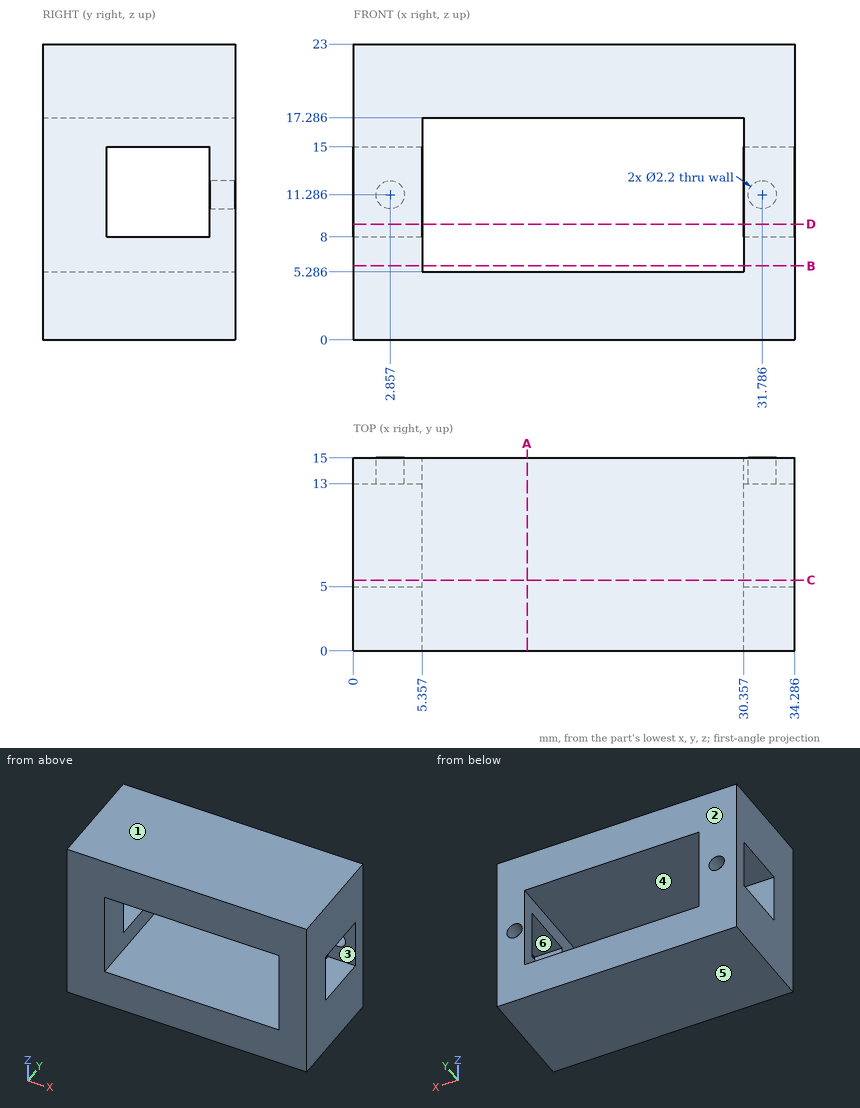
Design review of the part shown in the three views and the two pictorial views. Dimensions are in mm from the part's minimum x, y and z. A direction names the side the tool comes from. Round coordinates to 2 decimals unless told otherwise and drop trailing zeros. Loops run counter-clockwise (first coordinate to the right, second up) from the corner with the lowest first, then second, coordinate; pieces in that order, holes last. Notation, with made-up numbers: (-0.75, -38) -> (10.25, -38) arc R22 ccw to (10.25, -30) -> close; hole circle Ø2 at (14, -29). An arc over 180 degrees is marked (long way). Use one line per item in the form item = value. Start each with the question number.
Q1. For pin 1 Ø1.8 at (x, z) = (31.79, 11.29) entering from +Y, flat-tipped, find the tip position at first contact; note if it passes through.
Q2. Wall thickness on line 1 along Z through (x, y) = (14, 7.75); line 2 along Z through (x, y) = (33.5, 12.25); line 3 along X through (y, z) = (10, 15.75): over which ranges is each line inside the solid? List them lowest first. Write a range as [from, to].
Q3. We need section D-D on z = 9. Give the boundary of the cut face in (x, y), then the cut area to 3 significant figures.
Q4. Draft analysis for pull direction Y (two halves, no side actions). For the marked faces 1, 2 and 3, state which applies: +Y half, -Y half, draft (parallel to the pull), parting line (faces both ways), or undercut.
Q5. We need section B-B on z = 5.75. Give the boundary of the cut face in (x, y), then the cut area to 3 significant figures.
Q6. Machinability: for the marked faces 4, 5 and 6, which of the approach directions +Z, -Z, +X, -X, +Y, -Y give a long, thin tool a straight path to every point of the face, cutting with its end or side? Answer none if there is none.
Q7. We need section C-C on y = 5.5. Give the boundary of the cut face in (x, z).
Q8. We need section A-A on x = 13.5. Give the boundary of the cut face in (y, z), then the cut area to 3 significant figures.
Calculated:
q1.pin_1 = 5
q2.line_1 = [0, 5.29], [17.29, 23]
q2.line_2 = [0, 8], [15, 23]
q2.line_3 = [0, 5.36], [30.36, 34.29]
q3.outline = (0, 0) -> (5.36, 0) -> (5.36, 5) -> (0, 5) -> close; (0, 13) -> (5.36, 13) -> (5.36, 15) -> (0, 15) -> close; (30.36, 0) -> (34.29, 0) -> (34.29, 5) -> (30.36, 5) -> close; (30.36, 13) -> (34.29, 13) -> (34.29, 15) -> (30.36, 15) -> close
q3.area = 65.0 mm²
q4.face_1 = draft
q4.face_2 = +Y half
q4.face_3 = undercut
q5.outline = (0, 0) -> (5.36, 0) -> (5.36, 15) -> (0, 15) -> close; (30.36, 0) -> (34.29, 0) -> (34.29, 15) -> (30.36, 15) -> close
q5.area = 139 mm²
q6.face_4 = +Y, -Y
q6.face_5 = -Z, +X, -X, +Y, -Y
q6.face_6 = +X, -X
q7.outline = (0, 0) -> (34.29, 0) -> (34.29, 8) -> (30.36, 8) -> (30.36, 5.29) -> (5.36, 5.29) -> (5.36, 8) -> (0, 8) -> close; (0, 15) -> (5.36, 15) -> (5.36, 17.29) -> (30.36, 17.29) -> (30.36, 15) -> (34.29, 15) -> (34.29, 23) -> (0, 23) -> close
q8.outline = (0, 0) -> (15, 0) -> (15, 5.29) -> (0, 5.29) -> close; (0, 17.29) -> (15, 17.29) -> (15, 23) -> (0, 23) -> close
q8.area = 165 mm²
